Geometry check sheet. Reference: drawing and pictorial views, mm from the part's lowest x, y, z. A direction names the side the tool comes from. Coordinates: 2 decimals unless noted, no trailing zeros. Write each loop counter-clockwise with the first axis right and the second up, starting at its lowest first coordinate (ties: lowest second). Pieces come first, ordered by that corner, then holes. Notation, with made-up numbers: (-37.75, 80.25) - (-29.75, 80.25) arc R22 cw to (-29.75, 108.25) - close; hole circle Ø3 at (-26.75, 31.25). An arc over 180 degrees is marked (long way). Use one line per item in the form item = value. Start each with the question number.
(1) Sectioned sample at B-B (y = 10). Record the cut outline in (x, z), and give its area (3 significant figures).
(2) Sectioned sample at D-D (z = 7.5). Record the cut outline in (x, y), and give its area (3 significant figures).
(3) Sectioned sample at C-C (x = 45). Record the cut outline in (y, z), and give its area (3 significant figures).
(4) Gauge pin test, flat ends, axial feed: pin 1 Ø3 at (x, y) = (23, 9.5) entering from +Z; pin 2 Ø4 at (x, y) = (5, 10) entering from -Z; pin 3 Ø3 at (x, y) = (5, 10) entering from -Z. Record the tip position at first contact, or that the pin passes through.
(5) Material ranges on line 1 (X direction, y = 10, z = 4.8); line 2 (X direction, y = 10, z = 10.25); line 3 (Y direction, x = 45, z = 5.45), recorded low to high. Write a range as [from, to].
(6) Mould release check, pull along Y, two halves, no side actions. Record for the marked faces 1, 2, 3 and 4: released by +Y, released by -Y, zero draft, split by the parting line, or undercut.
(7) Sectioned sample at A-A (z = 13.75). Record the cut outline in (x, y).
(8) Tool access check on the marked faces 5, 6 and 7. Record the directions out of +Z, -Z, +X, -X, +Y, -Y that give a thin tool (end or side, any length) a straight path to the whole face; none if there is none.
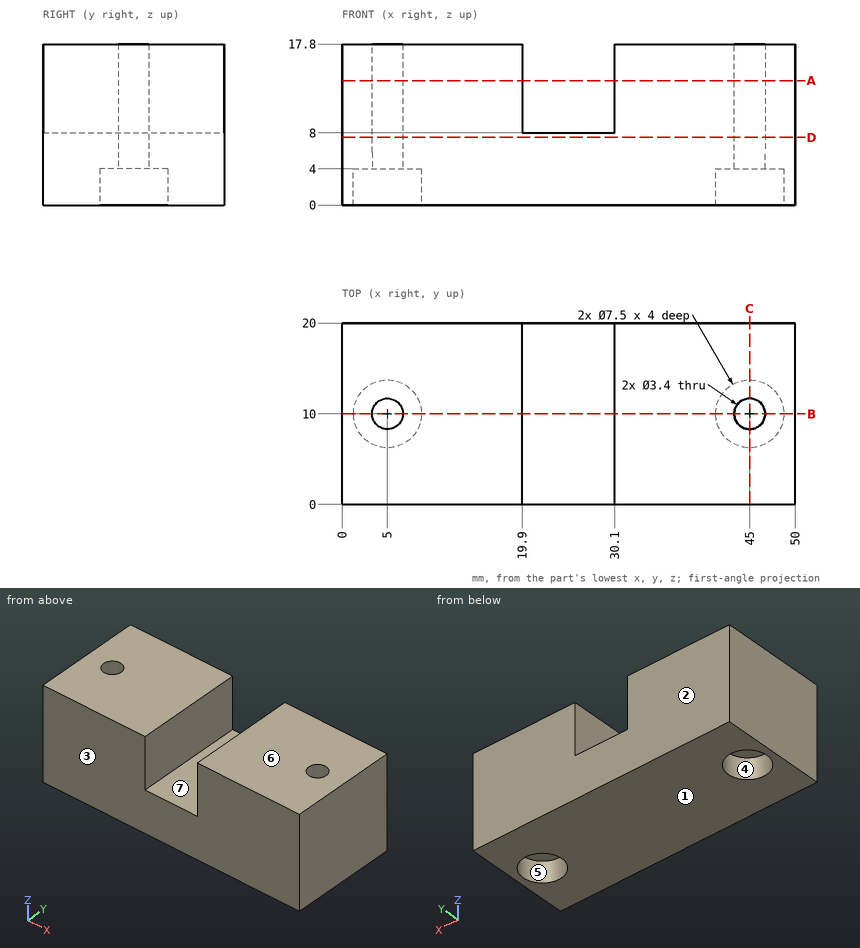
Answers below:
q1.outline = (0, 0) - (1.25, 0) - (1.25, 4) - (3.3, 4) - (3.3, 17.8) - (0, 17.8) - close; (6.7, 4) - (8.75, 4) - (8.75, 0) - (41.25, 0) - (41.25, 4) - (43.3, 4) - (43.3, 17.8) - (30.1, 17.8) - (30.1, 8) - (19.9, 8) - (19.9, 17.8) - (6.7, 17.8) - close; (46.7, 4) - (48.75, 4) - (48.75, 0) - (50, 0) - (50, 17.8) - (46.7, 17.8) - close
q1.area = 636 mm2
q2.outline = (0, 0) - (50, 0) - (50, 20) - (0, 20) - close; hole circle Ø3.4 at (5, 10); hole circle Ø3.4 at (45, 10)
q2.area = 982 mm2
q3.outline = (0, 0) - (6.25, 0) - (6.25, 4) - (8.3, 4) - (8.3, 17.8) - (0, 17.8) - close; (11.7, 4) - (13.75, 4) - (13.75, 0) - (20, 0) - (20, 17.8) - (11.7, 17.8) - close
q3.area = 279 mm2
q4.pin_1 = 8
q4.pin_2 = 4
q4.pin_3 = through
q5.line_1 = [0, 3.3], [6.7, 43.3], [46.7, 50]
q5.line_2 = [0, 3.3], [6.7, 19.9], [30.1, 43.3], [46.7, 50]
q5.line_3 = [0, 8.3], [11.7, 20]
q6.face_1 = zero draft
q6.face_2 = released by +Y
q6.face_3 = released by -Y
q6.face_4 = undercut
q7.outline = (0, 0) - (19.9, 0) - (19.9, 20) - (0, 20) - close; (30.1, 0) - (50, 0) - (50, 20) - (30.1, 20) - close; hole circle Ø3.4 at (5, 10); hole circle Ø3.4 at (45, 10)
q8.face_5 = -Z
q8.face_6 = +Z, +X, -X, +Y, -Y
q8.face_7 = +Z, +Y, -Y
